Verification items for the finished model (mm, model axes). A direction names the side the tool comes from. Coordinates: 2 decimals unless noted, no trailing zeros. Write each loop counter-clockwise with the first axis right and the second up, starting at its lowest first coordinate (ties: lowest second). Pieces come first, ordered by that corner, then holes. Notation, with made-up numbers: (72, 20.25) -> (128, 20.25) arc R24 ccw to (128, 35.25) -> close; hole circle Ø8 at (-10, -5). An arc over 180 degrees is marked (long way). Use a Markdown table: item, result. Add a question column.
from build123d import *

# Parameters (mm, degrees)
ESQUISSE1_W             = 22.5
ESQUISSE1_H             = 20
BOSS_EXTRU_1_DEPTH      = 1.2
ESQUISSE2_R             = 8
BOSS_EXTRU_2_DEPTH      = 13.8
COQUE2_T                = -0.5
ESQUISSE3_R             = 1
ENL_V_MAT_EXTRU_1_DEPTH = 29.375992396
ESQUISSE4_R             = 0.5
ENL_V_MAT_EXTRU_2_DEPTH = 2.8
BOSS_EXTRU_3_DEPTH      = 2
SYM_TRIE1_START         = -1.2
SYM_TRIE1_OUTLINE_R     = 8
SYM_TRIE1_DEPTH         = 15
SYM_TRIE1_2_OUTLINE_W   = 22.5
SYM_TRIE1_2_OUTLINE_H   = 20
SYM_TRIE1_2_OUTLINE_R   = 0.5
SYM_TRIE1_2_OUTLINE_R_2 = 8
SYM_TRIE1_2_DEPTH       = 1.2
SYM_TRIE1_3_DEPTH       = 2
COQUE4_T                = -0.5


# Read off the part's stored shape, not the designer's step: Symétrie1
with BuildPart() as part:
    # Esquisse1 → Boss.-Extru.1 (new body)
    with BuildSketch(Plane.XY):
        with Locations((-11.25, 0.416666667)):
            Rectangle(ESQUISSE1_W, ESQUISSE1_H)
    extrude(amount=-BOSS_EXTRU_1_DEPTH)

    # Esquisse2 → Boss.-Extru.2 (add)
    with BuildSketch(Plane.XY):
        with Locations(Location((-13.5, 0, 0), (0, 0, 180))):
            Circle(ESQUISSE2_R)
    extrude(amount=BOSS_EXTRU_2_DEPTH)

    # Coque2
    coque2_openings = [part.faces().sort_by_distance(p)[0] for p in [
        (-13.5, 0, 13.8),
    ]]
    offset(amount=COQUE2_T, openings=coque2_openings, kind=Kind.INTERSECTION)

    # Esquisse3 → Enlèv. mat.-Extru.1 (cut, through all)
    with BuildSketch(Plane.XY):
        with Locations((-20.497748718, -7.838681671)):
            Circle(ESQUISSE3_R)
    extrude(amount=-ENL_V_MAT_EXTRU_1_DEPTH, mode=Mode.SUBTRACT)

    # Esquisse4 → Enlèv. mat.-Extru.2 (cut)
    with BuildSketch(Plane.XY):
        with Locations(Location((-3.75, -7.838681671, 0), (0, 0, 180))):
            Circle(ESQUISSE4_R)
        with Locations(Location((-1.875, -7.838681671, 0), (0, 0, 180))):
            Circle(ESQUISSE4_R)
    extrude(amount=-ENL_V_MAT_EXTRU_2_DEPTH, mode=Mode.SUBTRACT)

    # Esquisse5 → Boss.-Extru.3 (add)
    with BuildSketch(Plane.XY):
        with BuildLine():
            Line((0, 6.438889699), (-4.894980877, 6.438889699))
            ThreePointArc((-4.894980877, 6.438889699), (-6.394980877, 7.938889699), (-4.894980877, 9.438889699))
            Line((-4.894980877, 9.438889699), (0, 9.438889699))
            Line((0, 9.438889699), (0, 6.438889699))
        make_face()
    extrude(amount=BOSS_EXTRU_3_DEPTH)



with BuildPart() as body_2:
    # Symétrie1 outline → Symétrie1 (new body)
    with BuildSketch(Plane.XY.offset(SYM_TRIE1_START)):
        with Locations((13.5, 0)):
            Circle(SYM_TRIE1_OUTLINE_R)
    extrude(amount=SYM_TRIE1_DEPTH)


with BuildPart() as part_1:
    add(part.part)

    add(body_2.part)  # Sym_trie1 2 merges body 2
    # Sym_trie1 2 outline → Sym_trie1 2 (add)
    with BuildSketch(Plane.XY.offset(SYM_TRIE1_START)):
        with Locations((11.25, 0.416666667)):
            Rectangle(SYM_TRIE1_2_OUTLINE_W, SYM_TRIE1_2_OUTLINE_H)
        with Locations((1.875, -7.838681671)):
            Circle(SYM_TRIE1_2_OUTLINE_R, mode=Mode.SUBTRACT)
        with Locations((3.75, -7.838681671)):
            Circle(SYM_TRIE1_2_OUTLINE_R, mode=Mode.SUBTRACT)
        with Locations((13.5, 0)):
            Circle(SYM_TRIE1_2_OUTLINE_R_2, mode=Mode.SUBTRACT)
    extrude(amount=SYM_TRIE1_2_DEPTH)

    # Sym_trie1 3 outline → Sym_trie1 3 (add)
    with BuildSketch(Plane.XY):
        with BuildLine():
            Line((0, 9.438889699), (0, 6.438889699))
            Line((0, 6.438889699), (4.894980877, 6.438889699))
            ThreePointArc((4.894980877, 6.438889699), (6.394980877, 7.938889699), (4.894980877, 9.438889699))
            Line((4.894980877, 9.438889699), (0, 9.438889699))
        make_face()
    extrude(amount=SYM_TRIE1_3_DEPTH)

    # Coque4
    coque4_openings = [part_1.faces().sort_by_distance(p)[0] for p in [
        (13.5, 0, 13.8),
    ]]
    offset(amount=COQUE4_T, openings=coque4_openings, kind=Kind.INTERSECTION)


solid = part_1.part
1) Cross-section at B-B on x = -3.75. Record the boundary of the cut face in (y, z).
2) Gauge pin test, flat ends, axial feed: pin 1 (1 mm diameter, centred on x = 13.5, z = 10, fed in from +Y); pin 2 (4 mm diameter, centred on x = 15.5, y = -4.5, fed in from +Z); pin 3 (0.6 mm diameter, centred on x = -0.5, z = 1, fed in from -Y). Record the tip position at first contact, or that the pin passes through.
3) Cross-section at A-A on x = 3.75. Record the boundary of the cut face in (y, z).
4) Cross-section at C-C on z = 1. Record the boundary of the cut face in (x, y), then the cut area to 3 significant figures.
5) Release check for a two-part mould opening along Y. For faces 4 (the face through (0, 8, 2)), 5 (the face through (5.895, 7.917, 0.486)), 6 (the face through (0, 9.439, 1)) record: released by +Y, released by -Y, zero draft, split by the parting line, or undercut.
6) Cross-section at D-D on y = 0. Record the boundary of the cut face in (x, z).
7) Set-up check for faces 1 (the face through (11, 1, -0.7)), 2 (the face through (0, -9.583, -1)), 3 (the face through (6.395, 7.906, 0.986)): record each of +Z, -Z, +X, -X, +Y, -Y from which the full face is reachable in a straight line by a thin tool's end or side.
8) Thickness scan on L1, parallel to Y at x = -3.75, z = -0.2; L2, parallel to Y at x = 13.5, z = 7.75; L3, parallel to Y at x = 3.75, z = -0.45. Record the ranges inside material, lowest first.
Returned:
| question | item | result |
|---|---|---|
| 1 | outline | (-9.58, -1.2) -> (-8.34, -1.2) -> (-8.34, -0.7) -> (-9.08, -0.7) -> (-9.08, -0.5) -> (-8.34, -0.5) -> (-8.34, 0) -> (-9.58, 0) -> close; (-7.34, -1.2) -> (10.42, -1.2) -> (10.42, 0) -> (9.44, 0) -> (9.44, 2) -> (6.44, 2) -> (6.44, 0) -> (-7.34, 0) -> (-7.34, -0.5) -> (9.92, -0.5) -> (9.92, -0.7) -> (-7.34, -0.7) -> close; hole (6.94, 0) -> (8.94, 0) -> (8.94, 1.5) -> (6.94, 1.5) -> close |
| 2 | pin 1 | stops at y = 8 |
| 2 | pin 2 | stops at z = -0.7 |
| 2 | pin 3 | stops at y = 6.44 |
| 3 | outline | (-9.58, -1.2) -> (-8.34, -1.2) -> (-8.34, 0) -> (-9.58, 0) -> close; (-7.34, -1.2) -> (10.42, -1.2) -> (10.42, 0) -> (9.44, 0) -> (9.44, 2) -> (6.44, 2) -> (6.44, 0) -> (-7.34, 0) -> close; hole (-9.08, -0.7) -> (-8.84, -0.7) -> (-8.84, -0.5) -> (-9.08, -0.5) -> close; hole (-6.84, -0.7) -> (9.92, -0.7) -> (9.92, -0.5) -> (8.94, -0.5) -> (8.94, 1.5) -> (6.94, 1.5) -> (6.94, -0.5) -> (-6.84, -0.5) -> close |
| 4 | outline | circle Ø16 at (-13.5, 0); (-4.89, 6.44) -> (4.89, 6.44) arc R1.5 ccw to (4.89, 9.44) -> (-4.89, 9.44) arc R1.5 ccw to start; circle Ø16 at (13.5, 0); hole circle Ø15 at (-13.5, 0); hole (-4.89, 6.94) -> (4.89, 6.94) arc R1 ccw to (4.89, 8.94) -> (-4.89, 8.94) arc R1 ccw to start; hole circle Ø15 at (13.5, 0) |
| 4 | area | 62.4 mm² |
| 5 | face 4 | zero draft |
| 5 | face 5 | undercut |
| 5 | face 6 | released by +Y |
| 6 | outline | (-22.5, -1.2) -> (22.5, -1.2) -> (22.5, 0) -> (21.5, 0) -> (21.5, 13.8) -> (21, 13.8) -> (21, -0.5) -> (22, -0.5) -> (22, -0.7) -> (0, -0.7) -> (0, -0.5) -> (6, -0.5) -> (6, 13.8) -> (5.5, 13.8) -> (5.5, 0) -> (-5.5, 0) -> (-5.5, 13.8) -> (-6, 13.8) -> (-6, -0.5) -> (-0.5, -0.5) -> (-0.5, -0.7) -> (-22, -0.7) -> (-22, -0.5) -> (-21, -0.5) -> (-21, 13.8) -> (-21.5, 13.8) -> (-21.5, 0) -> (-22.5, 0) -> close |
| 7 | face 1 | none |
| 7 | face 2 | +Z, -Z, +X, -X, -Y |
| 7 | face 3 | +Z |
| 8 | L1 | y = -9.58 to -8.34, -7.34 to 10.42 |
| 8 | L2 | y = -8 to -7.5, 7.5 to 8 |
| 8 | L3 | y = -9.58 to -8.34, -7.34 to 6.94, 8.94 to 10.42 |
